from build123d import *

# Parameters (mm, degrees)
SKETCH1_W                   = 1066.8
SKETCH1_H                   = 333.375
BOSS_EXTRUDE1_DEPTH         = 3.175
SKETCH2_W                   = 929.64
SKETCH2_H                   = 92.075
BOSS_EXTRUDE2_DEPTH         = 3.175
F_1_4_0_25_DIAMETER_HOLE1_D = 6.35
FILLET1_R                   = 3.175
CUT_EXTRUDE1_DEPTH          = 4.175


with BuildPart() as part:
    # Sketch1 → Boss-Extrude1 (new body)
    with BuildSketch(Plane(origin=(0, 0, 0), x_dir=(1, 0, 0), z_dir=(0, 1, 0))):
        with Locations((533.4, 166.6875)):
            Rectangle(SKETCH1_W, SKETCH1_H)
    extrude(amount=BOSS_EXTRUDE1_DEPTH)

    # Sketch2 → Boss-Extrude2 (add)
    with BuildSketch(Plane(origin=(0, 3.175, 0), x_dir=(1, 0, 0), z_dir=(0, 1, 0))):
        with Locations((533.4, 379.4125)):
            Rectangle(SKETCH2_W, SKETCH2_H)
    extrude(amount=-BOSS_EXTRUDE2_DEPTH)

    # 1/4 (0.25) Diameter Hole1 (through all)
    with Locations(Plane(origin=(0, 0, 0), x_dir=(-1, 0, 0), z_dir=(0, -1, 0))):
        with Locations((-71.4375, 39.6875), (-228.6, 409.575), (-533.4, 409.575), (-838.2, 409.575), (-995.3625, 293.6875), (-995.3625, 39.6875), (-71.4375, 293.6875)):
            Hole(F_1_4_0_25_DIAMETER_HOLE1_D / 2)

    # Fillet1
    fillet1_edges = [part.edges().sort_by_distance(p)[0] for p in [
        (998.22, 1.5875, -333.375),
        (998.22, 1.5875, -425.45),
        (68.58, 1.5875, -425.45),
        (68.58, 1.5875, -333.375),
        (0, 1.5875, -333.375),
        (1066.8, 1.5875, -333.375),
        (1066.8, 1.5875, 0),
        (0, 1.5875, 0),
    ]]
    fillet(fillet1_edges, radius=FILLET1_R)

    # Sketch9 → Cut-Extrude1 (cut, through all)
    with BuildSketch(Plane.XZ):
        with BuildLine():
            Line((860.425, -390.525), (815.975, -390.525))
            ThreePointArc((815.975, -390.525), (800.1, -374.65), (815.975, -358.775))
            Line((815.975, -358.775), (860.425, -358.775))
            ThreePointArc((860.425, -358.775), (876.3, -374.65), (860.425, -390.525))
        make_face()
        with BuildLine():
            Line((555.625, -390.525), (511.175, -390.525))
            ThreePointArc((511.175, -390.525), (495.3, -374.65), (511.175, -358.775))
            Line((511.175, -358.775), (555.625, -358.775))
            ThreePointArc((555.625, -358.775), (571.5, -374.65), (555.625, -390.525))
        make_face()
        with BuildLine():
            Line((250.825, -390.525), (206.375, -390.525))
            ThreePointArc((206.375, -390.525), (190.5, -374.65), (206.375, -358.775))
            Line((206.375, -358.775), (250.825, -358.775))
            ThreePointArc((250.825, -358.775), (266.7, -374.65), (250.825, -390.525))
        make_face()
    extrude(amount=-CUT_EXTRUDE1_DEPTH, mode=Mode.SUBTRACT)


solid = part.part
Can you work these out from the model? Positions are in its coordinate system, mm. Give positions to 0.01 mm unless a question says otherwise; leave off trailing zeros. Write each loop counter-clockwise with the first axis right and the second up, starting at its lowest first coordinate (ties: lowest second). Pieces come first, ordered by that corner, then holes. Notation, with made-up numbers: M 24,40.5 L 54,40.5 A14 cw 54,46.5 Z; hole C 89,-29 d2. An arc over 180 degrees is marked long. Answer in a Markdown table with one row per item. Add a question column.
Item 1: Imagine slicing it at A-A, the plane z = -374.65. Write out the boundary of the cut face in (x, y) (3 decimals).
Item 2: Please list where these lines run through material, in increasing order: L1, parallel to Z at x = 838.2, y = 1.05 (3 decimals); L2, parallel to Z at x = 219, y = 2.7 (3 decimals); L3, parallel to X at y = 1.6, z = -295.
Item 3: For pin 1 Ø8.5 at (x, z) = (533.4, -409.575) entering from +Y (3 decimals); pin 2 Ø1.6 at (x, y) = (1026, 2) entering from -Z (3 decimals); pin 3 Ø1 at (y, z) = (1.5, -369) entering from -X, each with a flat end and sliding along its axis, tell me the tip position at first contact or that it passes through.
Item 4: Imagine slicing it at B-B, the plane y = 0.5. State how many separate pieces and enclosed holes the cut face has, plus the area to 3 significant figures.
Evaluation:
| question | item | result |
|---|---|---|
| 1 | outline | M 68.58,0 L 190.5,0 L 190.5,3.175 L 68.58,3.175 Z; M 266.7,0 L 495.3,0 L 495.3,3.175 L 266.7,3.175 Z; M 571.5,0 L 800.1,0 L 800.1,3.175 L 571.5,3.175 Z; M 876.3,0 L 998.22,0 L 998.22,3.175 L 876.3,3.175 Z |
| 2 | L1 | z = -425.45 to -412.75, -406.4 to -390.525, -358.775 to 0 |
| 2 | L2 | z = -425.45 to -390.525, -358.775 to 0 |
| 2 | L3 | x = 0 to 68.55, 74.33 to 992.47, 998.25 to 1066.8 |
| 3 | pin 1 | stops at y = 3.175 |
| 3 | pin 2 | stops at z = -333.375 |
| 3 | pin 3 | stops at x = 68.58 |
| 4 | separate pieces | 1 |
| 4 | enclosed holes | 10 |
| 4 | area | 434,000 mm² |
